Design review of the part built by this model. Coordinates are the model's own, in mm. A direction names the side the tool comes from. Give positions to 0.01 mm unless a question says otherwise; leave off trailing zeros. Loops run counter-clockwise (first coordinate to the right, second up) from the corner with the lowest first, then second, coordinate; pieces in that order, holes last. Notation, with made-up numbers: M 64.5,56 L 105.5,56 A21 cw 105.5,85 Z; hole C 70,3 d4. An arc over 180 degrees is marked long. Answer as CSV lines item,"result".
```python
from build123d import *

# Parameters (mm, degrees)
F0_R     = 17
F1_DEPTH = 38
F2_R     = 5
F4_R     = 19
F5_DEPTH = 1.5


with BuildPart() as f1:
    # F0 (on Top) → F1 (new body)
    with BuildSketch(Plane.XY):
        Circle(F0_R)
    extrude(amount=F1_DEPTH)

    # F2
    f2_edges = [f1.edges().sort_by_distance(p)[0] for p in [
        (-17, 0, 0),
    ]]
    fillet(f2_edges, radius=F2_R)

    # F4 (on offset) → F5 (join)
    with BuildSketch(Plane.XY.offset(37)):
        Circle(F4_R)
    extrude(amount=-F5_DEPTH)


solid = f1.part
```
1. For P1, Ø10, axis at x = -4.5, z = 24, coming from the -Y side; P2, Ø4, axis at x = -12.5, z = 10, coming from the +Y side; P3, Ø1.5, axis at y = -13.5, z = 11, coming from the -X side, all flat-tipped, find the tip position at first contact; note any pin that passes through.
Answer block:
P1,"y = -17"
P2,"y = 13.37"
P3,"x = -11.24"
2. We need section D-D, the plane z = 26. Write out the cut boundary in (x, y).
Answer block:
outline,"C 0,0 d34"
3. To check wall thickness, follow L1, parallel to Z at x = 4, y = -11.5; L2, parallel to Z at x = 15, y = -11.5; L3, parallel to Y at x = -12, z = 25. State the ranges of each line that lie inside material, in increasing order. Write a range as [from, to].
Answer block:
L1,"[0, 38]"
L2,"[35.5, 37]"
L3,"[-12.04, 12.04]"
4. We need section A-A, the plane y = 0. Write out the cut boundary in (x, z), plus the area to 3 significant figures.
Answer block:
outline,"M -19,35.5 L -17,35.5 L -17,5 A5 ccw -12,0 L 12,0 A5 ccw 17,5 L 17,35.5 L 19,35.5 L 19,37 L 17,37 L 17,38 L -17,38 L -17,37 L -19,37 Z"
area,"1,290 mm²"
5. For faces 1 (the cylindrical face through (9.139, 14.334, 37.493)), 2 (the flat face through (0, 0, 38)), 3 (the flat face through (-14, -10, 35.5)), list the 3-axis set-ups (+Z, -Z, +X, -X, +Y, -Y) from which the entire face can be reached by the end or side of a thin tool; tool diameter is ignored.
Answer block:
face 1,"+Z"
face 2,"+Z, +X, -X, +Y, -Y"
face 3,"-Z"
6. We need section C-C, the plane z = 2. Write out the cut boundary in (x, y), plus the area to 3 significant figures.
Answer block:
outline,"C 0,0 d32"
area,"804 mm²"
